For this review, use the dimensioned drawing (mm, ordinates from the lowest corner) and the shaded views. A direction names the side the tool comes from. Coordinates: 2 decimals unless noted, no trailing zeros. Write each loop counter-clockwise with the first axis right and the second up, starting at its lowest first coordinate (ties: lowest second). Pieces come first, ordered by that corner, then holes. Notation, with made-up numbers: (-5.5, 5.25) - (32.5, 5.25) arc R28 cw to (32.5, 41.25) - close; hole circle Ø2 at (81, -18.75). An arc over 180 degrees is marked (long way). Use one line per item in the form item = value. Start each with the question number.
1) We need section C-C (y = 33). Give the boundary of the cut face in (x, z).
2) Mouldability with a two-part tool opening along Y and no side actions: class the marked faces 3, 4, 5 and 6 as pulls with the +Y half, pulls with the -Y half, needs draft (parallel to the pull), parting line crosses it, or undercut.
3) We need section D-D (x = 16.5). Give the boundary of the cut face in (y, z), plus the area to 4 significant figures.
4) Insertion check: P1, Ø1, axis at y = 31, z = 4, coming from the -X side; P2, Ø6, axis at x = 16.5, y = 33, coming from the -Z side; P3, Ø2.5, axis at x = 4, z = 2.5, coming from the -Y side; P4, Ø2.5, axis at y = 7, z = 3.5, coming from the -X side. Each pin has a flat end and moves straight along its axis. Give the tip position at first contact, or say it passes through.
5) We need section A-A (x = 24.5). Give the boundary of the cut face in (y, z), plus the area to 3 significant figures.
6) Tool access review of the marked faces 1 and 2: name each direction out of +Z, -Z, +X, -X, +Y, -Y from which nothing blocks a thin tool from reaching the whole face with its end or side.
7) We need section B-B (z = 4.5). Give the boundary of the cut face in (x, y).
8) For L1, parallel to Y at x = 16.5, z = 4.75; L2, parallel to Y at x = 16, z = 6.25; L3, parallel to X at y = 4, z = 2.5, list the stretches that pass through material, from the lowest coordinate up. Write a range as from..to.
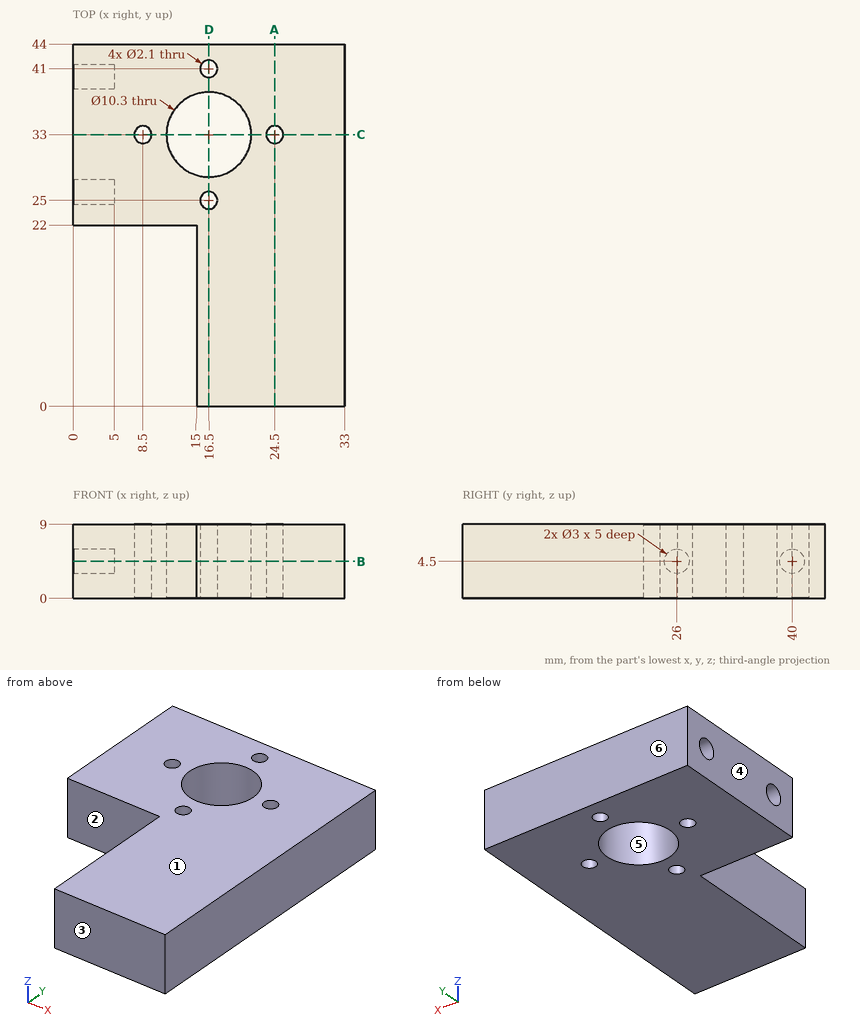
Determined:
q1.outline = (0, 0) - (7.45, 0) - (7.45, 9) - (0, 9) - close; (9.55, 0) - (11.35, 0) - (11.35, 9) - (9.55, 9) - close; (21.65, 0) - (23.45, 0) - (23.45, 9) - (21.65, 9) - close; (25.55, 0) - (33, 0) - (33, 9) - (25.55, 9) - close
q2.face_3 = pulls with the -Y half
q2.face_4 = needs draft
q2.face_5 = undercut
q2.face_6 = pulls with the +Y half
q3.outline = (0, 0) - (23.95, 0) - (23.95, 9) - (0, 9) - close; (26.05, 0) - (27.85, 0) - (27.85, 9) - (26.05, 9) - close; (38.15, 0) - (39.95, 0) - (39.95, 9) - (38.15, 9) - close; (42.05, 0) - (44, 0) - (44, 9) - (42.05, 9) - close
q3.area = 265.5 mm²
q4.P1 = 0
q4.P2 = through
q4.P3 = 22
q4.P4 = 15
q5.outline = (0, 0) - (31.95, 0) - (31.95, 9) - (0, 9) - close; (34.05, 0) - (44, 0) - (44, 9) - (34.05, 9) - close
q5.area = 377 mm²
q6.face_1 = +Z, +X, -X, +Y, -Y
q6.face_2 = +Z, -Z, -X, -Y
q7.outline = (0, 22) - (15, 22) - (15, 0) - (33, 0) - (33, 44) - (0, 44) - (0, 41.5) - (5, 41.5) - (5, 38.5) - (0, 38.5) - (0, 27.5) - (5, 27.5) - (5, 24.5) - (0, 24.5) - close; hole circle Ø2.1 at (8.5, 33); hole circle Ø10.3 at (16.5, 33); hole circle Ø2.1 at (16.5, 25); hole circle Ø2.1 at (16.5, 41); hole circle Ø2.1 at (24.5, 33)
q8.L1 = 0..23.95, 26.05..27.85, 38.15..39.95, 42.05..44
q8.L2 = 0..24.08, 25.92..27.87, 38.13..40.08, 41.92..44
q8.L3 = 15..33
